from build123d import *

# Parameters (mm, degrees)
F0_W     = 125
F0_H     = 75
F1_DEPTH = 70
F2_W     = 70
F2_H     = 25
F3_DEPTH = 70.001
F5_DEPTH = 75.001


with BuildPart() as f1:
    # F0 (on Front) → F1 (new body)
    with BuildSketch(Plane.XZ):
        with Locations((62.5, 37.5)):
            Rectangle(F0_W, F0_H)
    extrude(amount=F1_DEPTH)

    # F2 (on face) → F3 (cut, through all)
    with BuildSketch(Plane.XZ.offset(70)):
        with Locations((60, 62.5)):
            Rectangle(F2_W, F2_H)
    extrude(amount=-F3_DEPTH, mode=Mode.SUBTRACT)

    # F4 (on Top) → F5 (cut, through all)
    with BuildSketch(Plane.XY):
        Polygon((105, -118.377747), (105, -70), (105, -40), (70, -40), (70, -30), (45, -30), (45, -45), (0, -45), (0, -118.377747), align=None)
    extrude(amount=F5_DEPTH, mode=Mode.SUBTRACT)


solid = f1.part
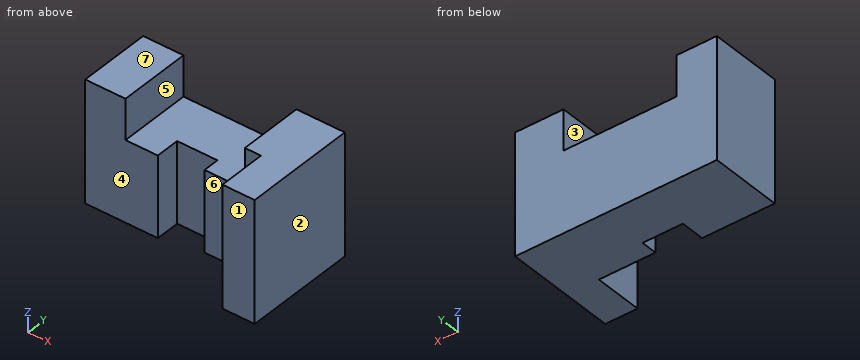
Part model, mm, in its own coordinate system. Face numbers are marked on the shaded views. A direction names the side the tool comes from. Coordinates: 2 decimals unless noted, no trailing zeros. Write each loop counter-clockwise with the first axis right and the second up, starting at its lowest first coordinate (ties: lowest second). Pieces come first, ordered by that corner, then holes. Notation, with made-up numbers: (-10.5, -38) - (28.5, -38) arc R15 ccw to (28.5, -16) - close; hole circle Ø2 at (-19, -11.75). An arc over 180 degrees is marked (long way). Put each result on its own line as item: value.
1. Two-plate mould, pull along X, no slides. Class the marked faces 1, 2 and 3: +X half, -X half, draft (parallel to the pull), parting line (faces both ways), or undercut.
Final values:
face 1: draft
face 2: +X half
face 3: undercut
2. 3-axis set-ups, long thin cutter, end or side, ignore diameter. For the marked faces 4, 5, 6 and 7: which of +Z, -Z, +X, -X, +Y, -Y reach the whole face in a straight line?
Final values:
face 4: +Z, -Z, -X, -Y
face 5: +Z, +Y, -Y
face 6: +Z, -Z, -Y
face 7: +Z, +X, -X, +Y, -Y
3. Band-saw the part on C-C (y = -5.5). Write the cut outline in (x, z).
Final values:
outline: (0, 0) - (125, 0) - (125, 75) - (95, 75) - (95, 50) - (25, 50) - (25, 75) - (0, 75) - close
4. Band-saw the part on A-A (y = -35.5). Write the cut outline in (x, z), then the cut area to 4 significant figures.
Final values:
outline: (0, 0) - (45, 0) - (45, 50) - (25, 50) - (25, 75) - (0, 75) - close; (70, 0) - (125, 0) - (125, 75) - (95, 75) - (95, 50) - (70, 50) - close
area: 6,375 mm²
5. Band-saw the part on B-B (z = 66). Write the cut outline in (x, y), then the cut area to 4 significant figures.
Final values:
outline: (0, -45) - (25, -45) - (25, 0) - (0, 0) - close; (95, -40) - (105, -40) - (105, -70) - (125, -70) - (125, 0) - (95, 0) - close
area: 2,925 mm²
6. Probe line 1 along X through (y, z) = (-19, 53); line 2 along Y through (x, z) = (35, 30); line 3 along X through (y, z) = (-54.5, 23.5). List the from-to ranges inside material, lowest first. Write a range as [from, to].
Final values:
line 1: x = [0, 25], [95, 125]
line 2: y = [-45, 0]
line 3: x = [105, 125]
7. Band-saw the part on D-D (z = 39). Write the cut outline in (x, y).
Final values:
outline: (0, -45) - (45, -45) - (45, -30) - (70, -30) - (70, -40) - (105, -40) - (105, -70) - (125, -70) - (125, 0) - (0, 0) - close
8. Flat gauge pins, fed straight in: pin 1 Ø1.5 at (x, z) = (18, 26.5) entering from -Y; pin 2 Ø5 at (x, y) = (90.5, -18) entering from +Z; pin 3 Ø20 at (x, z) = (59, 14.5) entering from -Y. Where does each tip first touch, or does it go through?
Final values:
pin 1: stops at y = -45
pin 2: stops at z = 50
pin 3: stops at y = -30
